Geometry: final body of the model. Coordinates: model frame, mm. Give positions to 0.01 mm unless a question says otherwise; leave off trailing zeros. Write each loop counter-clockwise with the first axis right and the second up, starting at its lowest first coordinate (ties: lowest second). Pieces come first, ordered by that corner, then holes. Notation, with made-up numbers: M 35,17.25 L 83,17.25 A20 ccw 83,30.25 Z; hole C -19,69 d5. An arc over 180 degrees is marked long. Answer as a JSON object with one key per item and string values.
from build123d import *

# Parameters (mm, degrees)
SKETCH_1_R          = 1.35
SKETCH_1_W          = 29.2
SKETCH_1_H          = 55.7
EXTRUDE_1_DEPTH     = 2
FILLET_1_R          = 1
CUT_EXTRUDE_2_REACH = 111.266
SKETCH_2_R          = 1.35
CUT_EXTRUDE_3_REACH = 111.266
CHAMFER_1_SIZE      = 5
CUT_EXTRUDE_4_REACH = 111.266
SKETCH_4_R          = 1.35
SKETCH_5_R          = 1.6
EXTRUDE_2_DEPTH     = 2
FILLET_3_R          = 10


with BuildPart() as part:
    # 草图1 → 凸台-拉伸1 (new body)
    with BuildSketch(Plane.XY):
        Polygon((-46.1, 41.813362069), (7.9, 41.813362069), (47.9, 41.813362069), (47.9, -98.186637931), (-46.1, -98.186637931), align=None)
        with Locations((-4.5, -95.186637931)):
            Circle(SKETCH_1_R, mode=Mode.SUBTRACT)
        with Locations((-24.5, -95.186637931)):
            Circle(SKETCH_1_R, mode=Mode.SUBTRACT)
        with Locations(Location((35.5, -95.186637931, 0), (0, 0, 180))):
            Circle(SKETCH_1_R, mode=Mode.SUBTRACT)
        with Locations((-29.8, 5.713362069)):
            Circle(SKETCH_1_R, mode=Mode.SUBTRACT)
        with Locations((-29.8, -16.286637931)):
            Circle(SKETCH_1_R, mode=Mode.SUBTRACT)
        with Locations(Location((4.8, -16.286637931, 0), (0, 0, 180))):
            Circle(SKETCH_1_R, mode=Mode.SUBTRACT)
        with Locations(Location((4.8, 5.713362069, 0), (0, 0, 180))):
            Circle(SKETCH_1_R, mode=Mode.SUBTRACT)
        with Locations(Location((4.8, 27.713362069, 0), (0, 0, 180))):
            Circle(SKETCH_1_R, mode=Mode.SUBTRACT)
        with Locations((-29.8, 27.713362069)):
            Circle(SKETCH_1_R, mode=Mode.SUBTRACT)
        with Locations(Location((15.5, -95.186637931, 0), (0, 0, 180))):
            Circle(SKETCH_1_R, mode=Mode.SUBTRACT)
        with Locations((-12.5, 8.963362069)):
            Rectangle(SKETCH_1_W, SKETCH_1_H, mode=Mode.SUBTRACT)
    extrude(amount=EXTRUDE_1_DEPTH)

    # 圆角1
    fillet_1_edges = [part.edges().sort_by_distance(p)[0] for p in [
        (-27.1, 36.813362069, 1),
        (-27.1, -18.886637931, 1),
        (2.1, -18.886637931, 1),
        (2.1, 36.813362069, 1),
    ]]
    fillet(fillet_1_edges, radius=FILLET_1_R)

    # 草图2 → 切除-拉伸2 (cut, up to next)
    with BuildSketch(Plane.XY.offset(2), mode=Mode.PRIVATE) as cut_extrude_2_sk1:
        with Locations((-42.1, 31.813362069)):
            Circle(SKETCH_2_R)
    cut_extrude_2_tool1 = extrude(cut_extrude_2_sk1.sketch, amount=-CUT_EXTRUDE_2_REACH, mode=Mode.PRIVATE) & part.part
    # 草图2 → 切除-拉伸2 (cut, up to next)
    with BuildSketch(Plane.XY.offset(2), mode=Mode.PRIVATE) as cut_extrude_2_sk2:
        with Locations((-42.1, 14.813362069)):
            Circle(SKETCH_2_R)
    cut_extrude_2_tool2 = extrude(cut_extrude_2_sk2.sketch, amount=-CUT_EXTRUDE_2_REACH, mode=Mode.PRIVATE) & part.part
    # 草图2 → 切除-拉伸2 (cut, up to next)
    with BuildSketch(Plane.XY.offset(2), mode=Mode.PRIVATE) as cut_extrude_2_sk3:
        with Locations(Location((-42.1, -71.186637931, 0), (0, 0, 180))):
            Circle(SKETCH_2_R)
    cut_extrude_2_tool3 = extrude(cut_extrude_2_sk3.sketch, amount=-CUT_EXTRUDE_2_REACH, mode=Mode.PRIVATE) & part.part
    # 草图2 → 切除-拉伸2 (cut, up to next)
    with BuildSketch(Plane.XY.offset(2), mode=Mode.PRIVATE) as cut_extrude_2_sk4:
        with Locations(Location((-42.1, -88.186637931, 0), (0, 0, 180))):
            Circle(SKETCH_2_R)
    cut_extrude_2_tool4 = extrude(cut_extrude_2_sk4.sketch, amount=-CUT_EXTRUDE_2_REACH, mode=Mode.PRIVATE) & part.part
    # 草图2 → 切除-拉伸2 (cut, up to next)
    with BuildSketch(Plane.XY.offset(2), mode=Mode.PRIVATE) as cut_extrude_2_sk5:
        with Locations((43.9, -88.186637931)):
            Circle(SKETCH_2_R)
    cut_extrude_2_tool5 = extrude(cut_extrude_2_sk5.sketch, amount=-CUT_EXTRUDE_2_REACH, mode=Mode.PRIVATE) & part.part
    # 草图2 → 切除-拉伸2 (cut, up to next)
    with BuildSketch(Plane.XY.offset(2), mode=Mode.PRIVATE) as cut_extrude_2_sk6:
        with Locations((43.9, -71.186637931)):
            Circle(SKETCH_2_R)
    cut_extrude_2_tool6 = extrude(cut_extrude_2_sk6.sketch, amount=-CUT_EXTRUDE_2_REACH, mode=Mode.PRIVATE) & part.part
    # 草图2 → 切除-拉伸2 (cut, up to next)
    with BuildSketch(Plane.XY.offset(2), mode=Mode.PRIVATE) as cut_extrude_2_sk7:
        with Locations((43.9, 21.813362069)):
            Circle(SKETCH_2_R)
    cut_extrude_2_tool7 = extrude(cut_extrude_2_sk7.sketch, amount=-CUT_EXTRUDE_2_REACH, mode=Mode.PRIVATE) & part.part
    # 草图2 → 切除-拉伸2 (cut, up to next)
    with BuildSketch(Plane.XY.offset(2), mode=Mode.PRIVATE) as cut_extrude_2_sk8:
        with Locations((43.9, 4.813362069)):
            Circle(SKETCH_2_R)
    cut_extrude_2_tool8 = extrude(cut_extrude_2_sk8.sketch, amount=-CUT_EXTRUDE_2_REACH, mode=Mode.PRIVATE) & part.part
    add(cut_extrude_2_tool1.solids().sort_by_distance((-42.1, 31.813362, 2))[0], mode=Mode.SUBTRACT)
    add(cut_extrude_2_tool2.solids().sort_by_distance((-42.1, 14.813362, 2))[0], mode=Mode.SUBTRACT)
    add(cut_extrude_2_tool3.solids().sort_by_distance((-42.1, -71.186638, 2))[0], mode=Mode.SUBTRACT)
    add(cut_extrude_2_tool4.solids().sort_by_distance((-42.1, -88.186638, 2))[0], mode=Mode.SUBTRACT)
    add(cut_extrude_2_tool5.solids().sort_by_distance((43.9, -88.186638, 2))[0], mode=Mode.SUBTRACT)
    add(cut_extrude_2_tool6.solids().sort_by_distance((43.9, -71.186638, 2))[0], mode=Mode.SUBTRACT)
    add(cut_extrude_2_tool7.solids().sort_by_distance((43.9, 21.813362, 2))[0], mode=Mode.SUBTRACT)
    add(cut_extrude_2_tool8.solids().sort_by_distance((43.9, 4.813362, 2))[0], mode=Mode.SUBTRACT)

    # 草图3 → 切除-拉伸3 (cut, up to next)
    with BuildSketch(Plane.XY.offset(2), mode=Mode.PRIVATE) as cut_extrude_3_sk1:
        with BuildLine():
            Line((-3, -40.186637931), (-3, -76.186637931))
            ThreePointArc((-3, -76.186637931), (0, -79.186637931), (3, -76.186637931))
            Line((3, -76.186637931), (3, -40.186637931))
            ThreePointArc((3, -40.186637931), (0, -37.186637931), (-3, -40.186637931))
        make_face()
    cut_extrude_3_tool1 = extrude(cut_extrude_3_sk1.sketch, amount=-CUT_EXTRUDE_3_REACH, mode=Mode.PRIVATE) & part.part
    # 草图3 → 切除-拉伸3 (cut, up to next)
    with BuildSketch(Plane.XY.offset(2), mode=Mode.PRIVATE) as cut_extrude_3_sk2:
        with BuildLine():
            Line((12, -40.186637931), (12, -76.186637931))
            ThreePointArc((12, -76.186637931), (15, -79.186637931), (18, -76.186637931))
            Line((18, -76.186637931), (18, -40.186637931))
            ThreePointArc((18, -40.186637931), (15, -37.186637931), (12, -40.186637931))
        make_face()
    cut_extrude_3_tool2 = extrude(cut_extrude_3_sk2.sketch, amount=-CUT_EXTRUDE_3_REACH, mode=Mode.PRIVATE) & part.part
    # 草图3 → 切除-拉伸3 (cut, up to next)
    with BuildSketch(Plane.XY.offset(2), mode=Mode.PRIVATE) as cut_extrude_3_sk3:
        with BuildLine():
            Line((27, -40.186637931), (27, -76.186637931))
            ThreePointArc((27, -76.186637931), (30, -79.186637931), (33, -76.186637931))
            Line((33, -76.186637931), (33, -40.186637931))
            ThreePointArc((33, -40.186637931), (30, -37.186637931), (27, -40.186637931))
        make_face()
    cut_extrude_3_tool3 = extrude(cut_extrude_3_sk3.sketch, amount=-CUT_EXTRUDE_3_REACH, mode=Mode.PRIVATE) & part.part
    # 草图3 → 切除-拉伸3 (cut, up to next)
    with BuildSketch(Plane.XY.offset(2), mode=Mode.PRIVATE) as cut_extrude_3_sk4:
        with BuildLine():
            Line((-18, -40.186637931), (-18, -76.186637931))
            ThreePointArc((-18, -76.186637931), (-15, -79.186637931), (-12, -76.186637931))
            Line((-12, -76.186637931), (-12, -40.186637931))
            ThreePointArc((-12, -40.186637931), (-15, -37.186637931), (-18, -40.186637931))
        make_face()
    cut_extrude_3_tool4 = extrude(cut_extrude_3_sk4.sketch, amount=-CUT_EXTRUDE_3_REACH, mode=Mode.PRIVATE) & part.part
    # 草图3 → 切除-拉伸3 (cut, up to next)
    with BuildSketch(Plane.XY.offset(2), mode=Mode.PRIVATE) as cut_extrude_3_sk5:
        with BuildLine():
            Line((-33, -40.186637931), (-33, -76.186637931))
            ThreePointArc((-33, -76.186637931), (-30, -79.186637931), (-27, -76.186637931))
            Line((-27, -76.186637931), (-27, -40.186637931))
            ThreePointArc((-27, -40.186637931), (-30, -37.186637931), (-33, -40.186637931))
        make_face()
    cut_extrude_3_tool5 = extrude(cut_extrude_3_sk5.sketch, amount=-CUT_EXTRUDE_3_REACH, mode=Mode.PRIVATE) & part.part
    # 草图3 → 切除-拉伸3 (cut, up to next)
    with BuildSketch(Plane.XY.offset(2), mode=Mode.PRIVATE) as cut_extrude_3_sk6:
        with BuildLine():
            Line((16.4, -15.186637931), (31.4, -15.186637931))
            ThreePointArc((31.4, -15.186637931), (34.4, -18.186637931), (31.4, -21.186637931))
            Line((31.4, -21.186637931), (16.4, -21.186637931))
            ThreePointArc((16.4, -21.186637931), (13.4, -18.186637931), (16.4, -15.186637931))
        make_face()
    cut_extrude_3_tool6 = extrude(cut_extrude_3_sk6.sketch, amount=-CUT_EXTRUDE_3_REACH, mode=Mode.PRIVATE) & part.part
    # 草图3 → 切除-拉伸3 (cut, up to next)
    with BuildSketch(Plane.XY.offset(2), mode=Mode.PRIVATE) as cut_extrude_3_sk7:
        with BuildLine():
            Line((16.4, -0.186637931), (31.4, -0.186637931))
            ThreePointArc((31.4, -0.186637931), (34.4, -3.186637931), (31.4, -6.186637931))
            Line((31.4, -6.186637931), (16.4, -6.186637931))
            ThreePointArc((16.4, -6.186637931), (13.4, -3.186637931), (16.4, -0.186637931))
        make_face()
    cut_extrude_3_tool7 = extrude(cut_extrude_3_sk7.sketch, amount=-CUT_EXTRUDE_3_REACH, mode=Mode.PRIVATE) & part.part
    # 草图3 → 切除-拉伸3 (cut, up to next)
    with BuildSketch(Plane.XY.offset(2), mode=Mode.PRIVATE) as cut_extrude_3_sk8:
        with BuildLine():
            Line((16.4, 14.813362069), (31.4, 14.813362069))
            ThreePointArc((31.4, 14.813362069), (34.4, 11.813362069), (31.4, 8.813362069))
            Line((31.4, 8.813362069), (16.4, 8.813362069))
            ThreePointArc((16.4, 8.813362069), (13.4, 11.813362069), (16.4, 14.813362069))
        make_face()
    cut_extrude_3_tool8 = extrude(cut_extrude_3_sk8.sketch, amount=-CUT_EXTRUDE_3_REACH, mode=Mode.PRIVATE) & part.part
    add(cut_extrude_3_tool1.solids().sort_by_distance((0, -58.186638, 2))[0], mode=Mode.SUBTRACT)
    add(cut_extrude_3_tool2.solids().sort_by_distance((15, -58.186638, 2))[0], mode=Mode.SUBTRACT)
    add(cut_extrude_3_tool3.solids().sort_by_distance((30, -58.186638, 2))[0], mode=Mode.SUBTRACT)
    add(cut_extrude_3_tool4.solids().sort_by_distance((-15, -58.186638, 2))[0], mode=Mode.SUBTRACT)
    add(cut_extrude_3_tool5.solids().sort_by_distance((-30, -58.186638, 2))[0], mode=Mode.SUBTRACT)
    add(cut_extrude_3_tool6.solids().sort_by_distance((23.9, -18.186638, 2))[0], mode=Mode.SUBTRACT)
    add(cut_extrude_3_tool7.solids().sort_by_distance((23.9, -3.186638, 2))[0], mode=Mode.SUBTRACT)
    add(cut_extrude_3_tool8.solids().sort_by_distance((23.9, 11.813362, 2))[0], mode=Mode.SUBTRACT)

    # 倒角1
    chamfer_1_edges = [part.edges().sort_by_distance(p)[0] for p in [
        (-46.1, -98.186637931, 1),
        (-46.1, 41.813362069, 1),
        (47.9, -98.186637931, 1),
    ]]
    chamfer(chamfer_1_edges, length=CHAMFER_1_SIZE)

    # 草图4 → 切除-拉伸4 (cut, up to next)
    with BuildSketch(Plane.XY.offset(2), mode=Mode.PRIVATE) as cut_extrude_4_sk1:
        with Locations((11.479260953, 33.813362069)):
            Circle(SKETCH_4_R)
    cut_extrude_4_tool1 = extrude(cut_extrude_4_sk1.sketch, amount=-CUT_EXTRUDE_4_REACH, mode=Mode.PRIVATE) & part.part
    # 草图4 → 切除-拉伸4 (cut, up to next)
    with BuildSketch(Plane.XY.offset(2), mode=Mode.PRIVATE) as cut_extrude_4_sk2:
        with Locations((27.9, 29.413438302)):
            Circle(SKETCH_4_R)
    cut_extrude_4_tool2 = extrude(cut_extrude_4_sk2.sketch, amount=-CUT_EXTRUDE_4_REACH, mode=Mode.PRIVATE) & part.part
    # 草图4 → 切除-拉伸4 (cut, up to next)
    with BuildSketch(Plane.XY.offset(2), mode=Mode.PRIVATE) as cut_extrude_4_sk3:
        Polygon((3.000756209, 42.296827651), (53.432967786, 28.783557286), (46.405100875, 52.816513179), align=None)
    cut_extrude_4_tool3 = extrude(cut_extrude_4_sk3.sketch, amount=-CUT_EXTRUDE_4_REACH, mode=Mode.PRIVATE) & part.part
    add(cut_extrude_4_tool1.solids().sort_by_distance((11.479261, 33.813362, 2))[0], mode=Mode.SUBTRACT)
    add(cut_extrude_4_tool2.solids().sort_by_distance((27.9, 29.413438, 2))[0], mode=Mode.SUBTRACT)
    add(cut_extrude_4_tool3.solids().sort_by_distance((34.279608, 41.298966, 2))[0], mode=Mode.SUBTRACT)

    # 草图5 → 凸台-拉伸2 (add)
    with BuildSketch(Plane.XY.offset(2)):
        with BuildLine():
            Line((47.9, 30.266111536), (67.851828366, 50.217939902))
            ThreePointArc((67.851828366, 50.217939902), (68.053357953, 60.615045013), (57.67187216, 61.219331022))
            Line((57.67187216, 61.219331022), (27.798319678, 35.652340545))
            Line((27.798319678, 35.652340545), (25.855389408, 33.004755671))
            Line((25.855389408, 33.004755671), (41.831287437, 29.328293781))
            Line((41.831287437, 29.328293781), (47.9, 30.266111536))
        make_face()
        with Locations((62.548527507, 55.521240761)):
            Circle(SKETCH_5_R, mode=Mode.SUBTRACT)
    extrude(amount=-EXTRUDE_2_DEPTH)

    # 圆角3
    fillet_3_edges = [part.edges().sort_by_distance(p)[0] for p in [
        (47.9, 30.266111536, 1),
        (27.798319678, 35.652340545, 1),
    ]]
    fillet(fillet_3_edges, radius=FILLET_3_R)


solid = part.part
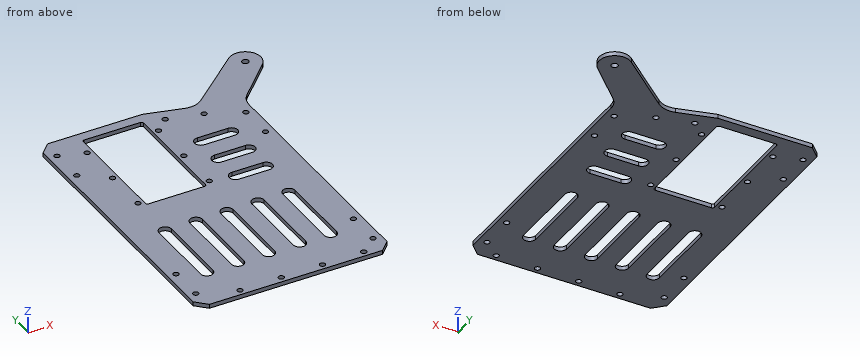
1) Contact query for flat-ended pins moving along their axis: P1, Ø2, axis at x = -25.5, y = -24.5, coming from the -Z side; P2, Ø1, axis at y = 5, z = 1.5, coming from the +X side; P3, Ø1.6, axis at x = 27.9, y = 29.41, coming from the +Z side. Output: stop coordinate, or through.
Geometry check:
{"P1": "stops at z = 0", "P2": "stops at x = 47.9", "P3": "passes through"}
2) Cut plane B-B on y = -81.5. Return loops of the section in (x, z), and give its area (3 significant figures).
Geometry check:
{"outline": "M -46.1,0 L 47.9,0 L 47.9,2 L -46.1,2 Z", "area": "188 mm2"}
3) Cut plane C-C on z = 0.6. Give the number of separate pieces and of enclosed holes in the cut face, and give its area (3 significant figures).
Geometry check:
{"separate pieces": "1", "enclosed holes": "30", "area": "10,200 mm2"}
4) Cut plane A-A on x = -20. Return loops of the section in (y, z), and give its area (3 significant figures).
Geometry check:
{"outline": "M -98.19,0 L -18.89,0 L -18.89,2 L -98.19,2 Z; M 36.81,0 L 41.81,0 L 41.81,2 L 36.81,2 Z", "area": "169 mm2"}
5) Line query: line 1 (X direction, y = -66, z = 1.7); line 2 (Y direction, x = 4.8, z = 0.6); line 3 (Y direction, x = -29.8, z = 1.2). Output: solid intervals per line, ascending. Write a range as from..to.
Geometry check:
{"line 1": "x = -46.1..-33, -27..-18, -12..-3, 3..12, 18..27, 33..47.9", "line 2": "y = -98.19..-17.64, -14.94..4.36, 7.06..26.36, 29.06..41.81", "line 3": "y = -98.19..-79.18, -37.19..-17.64, -14.94..4.36, 7.06..26.36, 29.06..41.81"}
